Check sheet for the modelled part. Datum: model origin and axes. Units: mm. A direction names the side the tool comes from. Coordinates: 2 decimals unless noted, no trailing zeros. Write each loop counter-clockwise with the first axis right and the second up, starting at its lowest first coordinate (ties: lowest second). Pieces come first, ordered by that corner, then holes. Notation, with made-up numbers: (26, 56.25) -> (74, 56.25) arc R22 cw to (74, 92.25) -> close; hole circle Ø1 at (-32, 16). An arc over 180 degrees is marked (long way). One line per item, written item: value. Start each with the question number.
1) Sectioned sample at A-A on z = 0. Enter the section's corners in (x, y) (3 decimals), plus the area to 3 significant figures.
2) Set-up check for faces 1 (the flat face through (-4, -8, 2)), 2 (the flat face through (-0.6, -6.094, 6.5)): record each of +Z, -Z, +X, -X, +Y, -Y from which the full face is reachable in a straight line by a thin tool's end or side.
3) Scan lines: line 1 along X through (y, z) = (2, 0) (3 decimals); line 2 along Y through (x, z) = (5.75, 5.5). Record each from-to range of solid material in increasing order. Write a range as [from, to].
4) Gauge pin test, flat ends, axial feed: P1, Ø2, axis at y = -3.5, z = 5.5, coming from the +X side; P2, Ø2, axis at x = 4, y = 5.5, coming from the -Z side; P3, Ø3, axis at y = 0, z = 6.5, coming from the -X side. Record the tip position at first contact, or that the pin passes through.
5) Sectioned sample at B-B on x = 0. Enter the section's corners in (y, z) (3 decimals).
6) Draft check along Z on faces 3 (the flat face through (-0.6, 3.556, 6.5)), 4 (the cylindrical face through (-5.051, -1.201, 3.873)), 5 (the cylindrical face through (-0.867, 0.112, 3.905)). Enter one of: +Z half, -Z half, draft (parallel to the pull), parting line (faces both ways), or undercut.
7) Sectioned sample at D-D on z = -6. Enter the section's corners in (x, y), plus the area to 3 significant figures.
8) Sectioned sample at C-C on y = -0.5. Enter the section's corners in (x, z) (3 decimals).
```python
from build123d import *

# Parameters (mm, degrees)
SKETCH1_R                = 8
BOSS_EXTRUDE1_DEPTH      = 8
BOSS_EXTRUDE1_DEPTH_BACK = 8
SKETCH2_R                = 8
SKETCH2_R_2              = 6.36499997
CUT_EXTRUDE1_DEPTH       = 3.556
CUT_EXTRUDE1_DEPTH_BACK  = 6.094
SKETCH3_R                = 4
CUT_EXTRUDE2_DEPTH       = 17


with BuildPart() as part:
    # Sketch1 → Boss-Extrude1 (new body, two sides)
    with BuildSketch(Plane(origin=(0, 0, 0), x_dir=(1, 0, 0), z_dir=(0, 1, 0))) as boss_extrude1_sk:
        Circle(SKETCH1_R)
    extrude(amount=BOSS_EXTRUDE1_DEPTH)
    extrude(boss_extrude1_sk.sketch, amount=-BOSS_EXTRUDE1_DEPTH_BACK)

    # Sketch2 → Cut-Extrude1 (cut, two sides)
    with BuildSketch(Plane(origin=(0, 0, 0), x_dir=(1, 0, 0), z_dir=(0, 1, 0))) as cut_extrude1_sk:
        Circle(SKETCH2_R)
        Circle(SKETCH2_R_2, mode=Mode.SUBTRACT)
    extrude(amount=CUT_EXTRUDE1_DEPTH, mode=Mode.SUBTRACT)
    extrude(cut_extrude1_sk.sketch, amount=-CUT_EXTRUDE1_DEPTH_BACK, mode=Mode.SUBTRACT)

    # Sketch3 → Cut-Extrude2 (cut, through all)
    with BuildSketch(Plane(origin=(0, 8, 0), x_dir=(1, 0, 0), z_dir=(0, 1, 0))):
        Circle(SKETCH3_R)
    extrude(amount=-CUT_EXTRUDE2_DEPTH, mode=Mode.SUBTRACT)


solid = part.part
```
Answers:
1. outline: (-8, -8) -> (-4, -8) -> (-4, 8) -> (-8, 8) -> (-8, 3.556) -> (-6.365, 3.556) -> (-6.365, -6.094) -> (-8, -6.094) -> close; (4, -8) -> (8, -8) -> (8, -6.094) -> (6.365, -6.094) -> (6.365, 3.556) -> (8, 3.556) -> (8, 8) -> (4, 8) -> close
1. area: 96.4 mm2
2. face 1: +Z, -Z, +X, -X, -Y
2. face 2: none
3. line 1: x = [-6.365, -4], [4, 6.365]
3. line 2: y = [-8, -6.09], [3.56, 8]
4. P1: stops at x = 4.5
4. P2: stops at z = -7.42
4. P3: stops at x = -3.94
5. outline: (-8, -8) -> (-6.094, -8) -> (-6.094, -6.365) -> (3.556, -6.365) -> (3.556, -8) -> (8, -8) -> (8, -4) -> (-8, -4) -> close; (-8, 4) -> (8, 4) -> (8, 8) -> (3.556, 8) -> (3.556, 6.365) -> (-6.094, 6.365) -> (-6.094, 8) -> (-8, 8) -> close
6. face 3: draft
6. face 4: parting line
6. face 5: undercut
7. outline: (-5.29, -8) -> (5.29, -8) -> (5.29, -6.09) -> (2.12, -6.09) -> (2.12, 3.56) -> (5.29, 3.56) -> (5.29, 8) -> (-5.29, 8) -> (-5.29, 3.56) -> (-2.12, 3.56) -> (-2.12, -6.09) -> (-5.29, -6.09) -> close
7. area: 108 mm2
8. outline: circle Ø12.73 at (0, 0); hole circle Ø8 at (0, 0)
